Geometry: see drawing. Coordinates: mm, zero at the bounding-box minimum. Give positions to 0.01 mm unless a question says otherwise; leave off trailing zeros. Loops run counter-clockwise (first coordinate to the right, second up) from the corner with the lowest first, then second, coordinate; pieces in that order, holes last. Notation, with made-up numbers: (31.5, 60) - (44.5, 60) arc R14 cw to (44.5, 67) - close; hole circle Ø2 at (-13, -30). An arc over 180 degrees is marked (long way). Use CSV: the item, a comma, the result in double quotes. Start each with the question number.
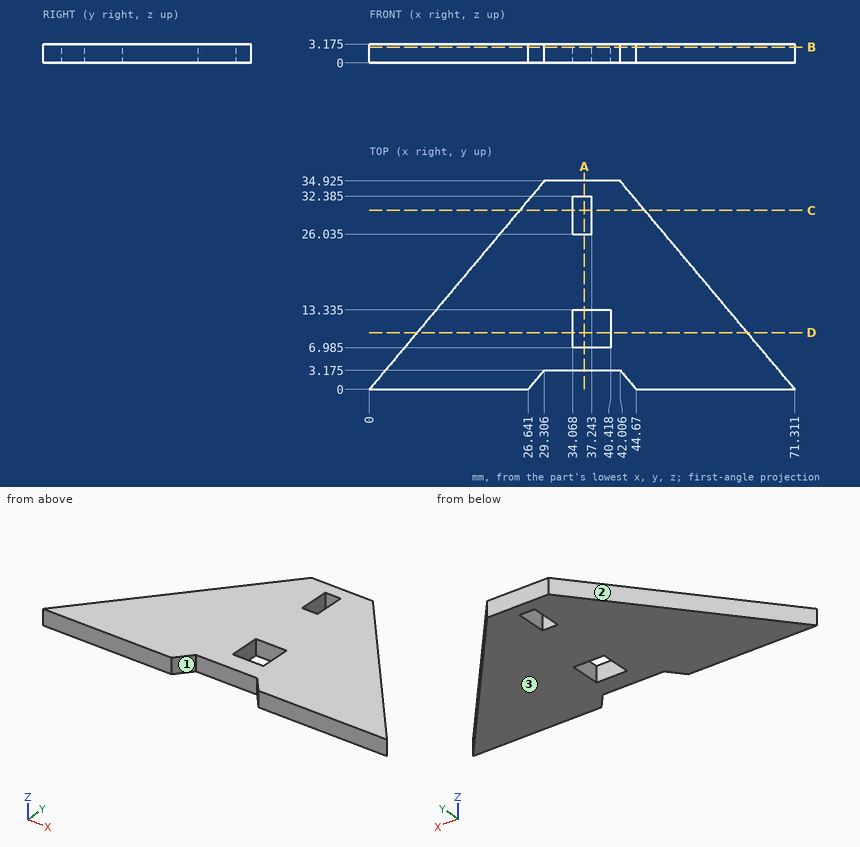
Item 1: Section D-D (y = 9.5). Output: boundary loops of the cut face in (x, z) (1 decimal), plus the area to 3 significant figures.
Item 2: Section B-B (z = 2.65). Output: boundary loops of the cut face in (x, y) (1 decimal).
Item 3: Section A-A (x = 36). Output: boundary loops of the cut face in (y, z) (1 decimal).
Item 4: Ray query, probe 1 along Y at (x, z) = (38, 1.3) (1 decimal); probe 2 along X at (y, z) = (27, 0.95) (1 decimal); probe 3 along X at (y, z) = (26.5, 2.4) (1 decimal). Return the intervals inside material, ascending.
Item 5: Section C-C (y = 30). Output: boundary loops of the cut face in (x, z) (1 decimal).
Item 6: Pin query (flat end, axial travel): pin 1 Ø1 at (x, z) = (37, 2) entering from -Y (3 decimals); pin 2 Ø8 at (x, y) = (54.5, 23.5) entering from +Z (3 decimals); pin 3 Ø5 at (x, y) = (14.5, 24.5) entering from -Z; pin 4 Ø1.6 at (y, z) = (28, 1) entering from +X. Return the tip coordinate at first contact, or that it passes through.
Item 7: Mould query, pull axis X, two halves, no side actions, for the marked faces 1, 2 and 3. Classes: pulls with the +X half, pulls with the -X half, needs draft (parallel to the pull), parting line crosses it, or undercut.
Outcome:
1,outline,"(8, 0) - (34.1, 0) - (34.1, 3.2) - (8, 3.2) - close; (40.4, 0) - (63.3, 0) - (63.3, 3.2) - (40.4, 3.2) - close"
1,area,"156 mm2"
2,outline,"(0, 0) - (26.6, 0) - (29.3, 3.2) - (42, 3.2) - (44.7, 0) - (71.3, 0) - (42, 34.9) - (29.3, 34.9) - close; hole (34.1, 7) - (40.4, 7) - (40.4, 13.3) - (34.1, 13.3) - close; hole (34.1, 26) - (37.2, 26) - (37.2, 32.4) - (34.1, 32.4) - close"
3,outline,"(3.2, 0) - (7, 0) - (7, 3.2) - (3.2, 3.2) - close; (13.3, 0) - (26, 0) - (26, 3.2) - (13.3, 3.2) - close; (32.4, 0) - (34.9, 0) - (34.9, 3.2) - (32.4, 3.2) - close"
4,probe 1,"y = 3.2 to 7, 13.3 to 34.9"
4,probe 2,"x = 22.7 to 34.1, 37.2 to 48.7"
4,probe 3,"x = 22.2 to 34.1, 37.2 to 49.1"
5,outline,"(25.2, 0) - (34.1, 0) - (34.1, 3.2) - (25.2, 3.2) - close; (37.2, 0) - (46.1, 0) - (46.1, 3.2) - (37.2, 3.2) - close"
6,pin 1,"stops at y = 3.175"
6,pin 2,"stops at z = 3.175"
6,pin 3,"passes through"
6,pin 4,"stops at x = 48.49"
7,face 1,"undercut"
7,face 2,"pulls with the -X half"
7,face 3,"needs draft"
